```python
from build123d import *

# Parameters (mm, degrees)
SKETCH002_R             = 5
PAD002_DEPTH            = 8
SKETCH003_R             = 6.7
PAD003_DEPTH            = 2.5
SKETCH004_R             = 1
PAD004_DEPTH            = 12
BODY001_PLACEMENT_ANGLE = 90


with BuildPart() as part:
    # Sketch002 → Pad002 (new body)
    with BuildSketch(Plane.XY):
        Circle(SKETCH002_R)
    extrude(amount=-PAD002_DEPTH)

    # Sketch003 → Pad003 (join)
    with BuildSketch(Plane.XY.offset(-5)):
        Circle(SKETCH003_R)
    extrude(amount=PAD003_DEPTH)

    # Sketch004 → Pad004 (join)
    with BuildSketch(Plane.XY):
        with Locations((2.5, 0)):
            Circle(SKETCH004_R)
        with Locations((-2.5, 0)):
            Circle(SKETCH004_R)
        with Locations((0, 2.5)):
            Circle(SKETCH004_R)
        with Locations((0, -2.5)):
            Circle(SKETCH004_R)
    extrude(amount=-PAD004_DEPTH)


with BuildPart() as part_1:
    # Body001 placement: moved
    add(part.part.moved(Location((55, 6, -7.5))).rotate(Axis((55, 6, -7.5), (0, 1, 0)), BODY001_PLACEMENT_ANGLE))


solid = part_1.part
```
Part model, mm, in its own coordinate system. A direction names the side the tool comes from. Give positions to 0.01 mm unless a question says otherwise; leave off trailing zeros. Order: outer loops, then holes, each group sorted by start corner. A loop starts at its lowest first (then second) coordinate and runs counter-clockwise, first axis right, second up. Notation, with made-up numbers: M -31,32 L 5,32 A9 ccw 5,40 Z; hole C 10.25,-4.75 d7. An arc over 180 degrees is marked long. Use a Markdown table: item, result. Add a question column.
(1) Saw through at C-C, the plane z = -10.75. Give the cut face in (x, y).
(2) 3-axis set-ups, long thin cutter, end or side, ignore diameter. For faces 5 (the face through (51.232, 3.434, -13.689)), 6 (the face through (48.52, 1.12, -6.42)): which of +Z, -Z, +X, -X, +Y, -Y reach the whole face in a straight line?
(3) Saw through at A-A, the plane x = 45.25. Give the cut face in (y, z), and give its area (3 significant figures).
(4) Saw through at D-D, the plane x = 48.75. Give the cut face in (y, z).
(5) Drop flat-ended pins along their axis: P1, Ø4, axis at x = 53.5, z = -5, coming from the +Y side; P2, Ø1, axis at x = 50, z = -12.5, coming from the +Y side; P3, Ø3, axis at x = 46.5, z = -4, coming from the +Y side. Give the stop position or say it passes through.
(6) Saw through at B-B, the plane y = 6. Give the cut face in (x, z), and give its area (4 significant figures).
(7) Probe line 1 along X through (y, z) = (7, -10.5); line 2 along X through (y, z) = (11.75, -7.5); line 3 along Z through (x, y) = (53.25, 8.5). List the from-to ranges inside material, lowest first. Write a range as [from, to].
(8) Mould opens along Y. For faces 1 (the face through (45.03, 9.49, -7.37)), 2 (the face through (45.028, 4.176, -6.763)), 3 (the face through (43, 6, -5)), 4 (the face through (53.77, 1.12, -6.42)) say: +Y half, -Y half, draft (parallel to the pull), parting line (faces both ways), or undercut.
Answer key:
| question | item | result |
|---|---|---|
| 1 | outline | M 43,5.34 L 47,5.34 L 47,2.2 L 50,2.2 L 50,0.14 L 52.5,0.14 L 52.5,2.2 L 55,2.2 L 55,9.8 L 52.5,9.8 L 52.5,11.86 L 50,11.86 L 50,9.8 L 47,9.8 L 47,6.66 L 43,6.66 Z |
| 2 | face 5 | +X, -X |
| 2 | face 6 | -X |
| 3 | outline | C 3.5,-7.5 d2; C 6,-10 d2; C 6,-5 d2; C 8.5,-7.5 d2 |
| 3 | area | 12.6 mm^2 |
| 4 | outline | C 6,-7.5 d10 |
| 5 | P1 | y = 12.66 |
| 5 | P2 | y = 10.96 |
| 5 | P3 | y = 10.54 |
| 6 | outline | M 43,-11 L 47,-11 L 47,-12.5 L 50,-12.5 L 50,-14.2 L 52.5,-14.2 L 52.5,-12.5 L 55,-12.5 L 55,-2.5 L 52.5,-2.5 L 52.5,-0.8 L 50,-0.8 L 50,-2.5 L 47,-2.5 L 47,-4 L 43,-4 L 43,-6 L 47,-6 L 47,-9 L 43,-9 Z |
| 6 | area | 104.5 mm^2 |
| 7 | line 1 | [47, 55] |
| 7 | line 2 | [50, 52.5] |
| 7 | line 3 | [-11.83, -3.17] |
| 8 | face 1 | undercut |
| 8 | face 2 | undercut |
| 8 | face 3 | draft |
| 8 | face 4 | parting line |
